Source: three-view drawing plus pictorial views. Frame: mm from the lowest corner of the part. Round coordinates to 2 decimals unless told otherwise and drop trailing zeros. Loops run counter-clockwise (first coordinate to the right, second up) from the corner with the lowest first, then second, coordinate; pieces in that order, holes last. Notation, with made-up numbers: (63.5, -33.5) -> (94.5, -33.5) arc R14 cw to (94.5, -26.5) -> close; hole circle Ø3 at (45, 88.5). An arc over 180 degrees is marked (long way). Answer as a JSON object with one key per item and string values. Group by question number.
Item 1: Section query A-A on x = 37.5. Return loops of the section in (y, z).
Item 2: Section query D-D on y = 3.55. Count the separate pieces of the cut face and the enclosed holes in it, and give its area (3 significant figures).
Item 3: Pin query (flat end, axial travel): pin 1 (1.5 mm diameter, centred on x = 10.5, y = 0.5, fed in from -Z). Return the tip coordinate at first contact, or that it passes through.
Item 4: Section query C-C on z = 10. Return loops of the section in (x, y).
Item 5: Material intervals for line 1 (Z direction, x = 10, y = 1.8); line 2 (X direction, y = 1.95, z = 10); line 3 (X direction, y = 4.15, z = 55), sorted ascending. Write a range as [from, to].
Item 6: Draft query along Z for the marked faces 1 and 2. Return one class per face: released by +Z, released by -Z, zero draft, split by the parting line, or undercut.
Item 7: Section query B-B on x = 10. Return loops of the section in (y, z), and give its area (3 significant figures).
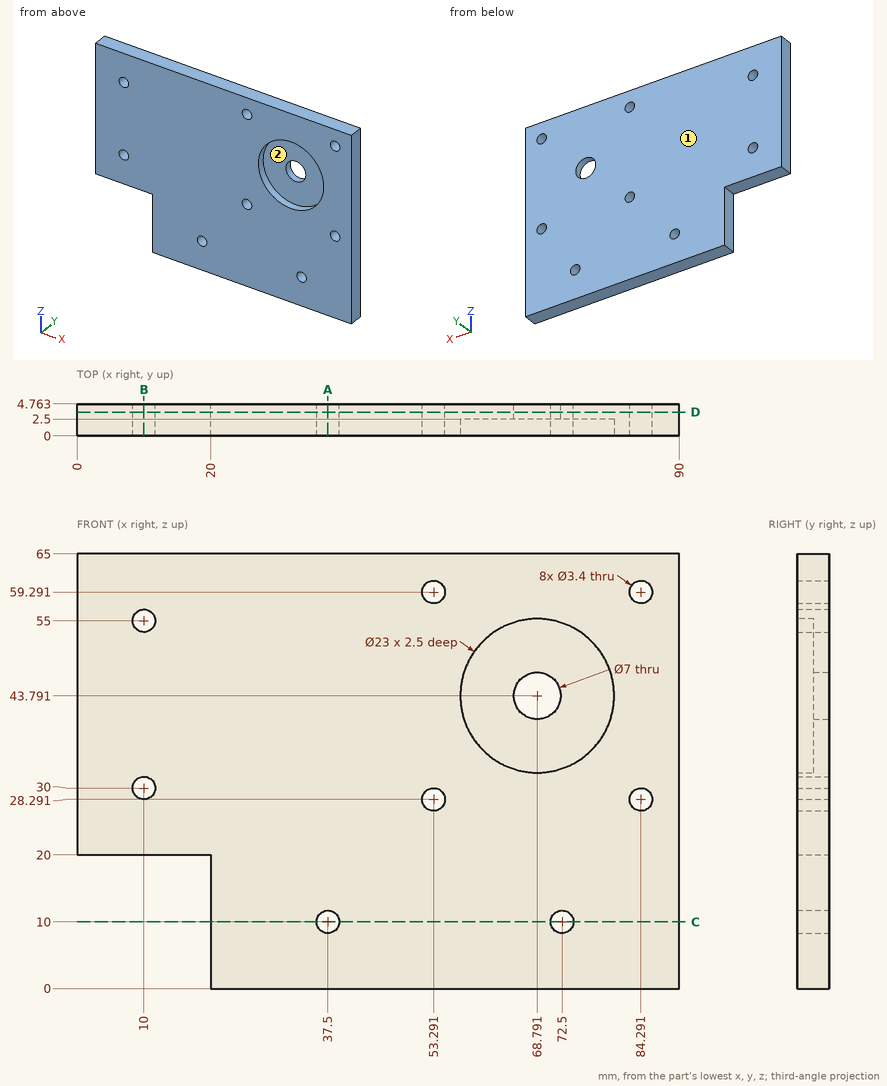
Solved:
{
 "1": {"outline": "(0, 0) -> (4.76, 0) -> (4.76, 8.3) -> (0, 8.3) -> close; (0, 11.7) -> (4.76, 11.7) -> (4.76, 65) -> (0, 65) -> close"},
 "2": {"separate pieces": "1", "enclosed holes": "9", "area": "5,340 mm²"},
 "3": {"pin 1": "z = 20"},
 "4": {"outline": "(20, 0) -> (35.8, 0) -> (35.8, 4.76) -> (20, 4.76) -> close; (39.2, 0) -> (70.8, 0) -> (70.8, 4.76) -> (39.2, 4.76) -> close; (74.2, 0) -> (90, 0) -> (90, 4.76) -> (74.2, 4.76) -> close"},
 "5": {"line 1": "[20, 28.3], [31.7, 53.3], [56.7, 65]", "line 2": "[20, 35.8], [39.2, 70.8], [74.2, 90]", "line 3": "[0, 8.3], [11.7, 90]"},
 "6": {"face 1": "zero draft", "face 2": "undercut"},
 "7": {"outline": "(0, 20) -> (4.76, 20) -> (4.76, 28.3) -> (0, 28.3) -> close; (0, 31.7) -> (4.76, 31.7) -> (4.76, 53.3) -> (0, 53.3) -> close; (0, 56.7) -> (4.76, 56.7) -> (4.76, 65) -> (0, 65) -> close", "area": "182 mm²"}
}
